Verification items for this drawing (mm, ordinates from the low corner). Give positions to 0.01 mm unless a question says otherwise; leave off trailing zeros. Order: outer loops, then holes, each group sorted by start corner. A loop starts at its lowest first (then second) coordinate and runs counter-clockwise, first axis right, second up. Notation, with made-up numbers: M 54.5,43.25 L 58.5,43.25 A23 cw 58.5,69.25 Z; hole C 12,52.5 d1. An arc over 180 degrees is marked long. Return JSON: item names as keys, results as strings. Group by question number.
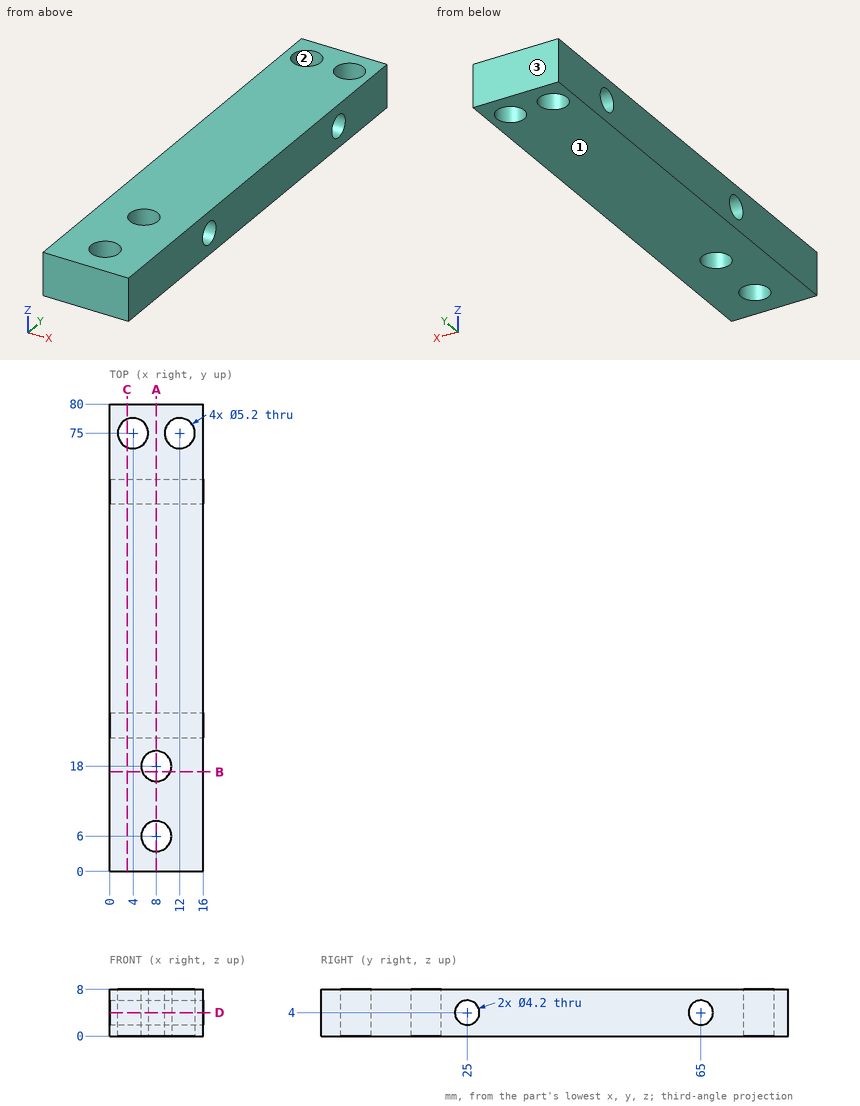
1) Sectioned sample at C-C on x = 3. Record the boundary of the cut face in (y, z).
2) Sectioned sample at D-D on z = 4. Record the boundary of the cut face in (x, y), then the cut area to 3 significant figures.
3) Release check for a two-part mould opening along Y. For the marked faces 1, 2 and 3 record: released by +Y, released by -Y, zero draft, split by the parting line, or undercut.
4) Sectioned sample at A-A on x = 8. Record the boundary of the cut face in (y, z).
5) Material ranges on line 1 along Z through (x, y) = (11.75, 25); line 2 along X through (y, z) = (73, 1.5); line 3 along Y through (x, z) = (14.75, 3.5), recorded low to high.
6) Sectioned sample at B-B on y = 17. Record the boundary of the cut face in (x, z), then the cut area to 3 significant figures.
7) Depth check by flat-ended pin: P1, Ø4, axis at x = 8, y = 6, coming from the -Z side. Enter the tip coordinate at first touch or a pass-through.
Reply:
{
 "1": {"outline": "M 0,0 L 72.6,0 L 72.6,8 L 0,8 Z; M 77.4,0 L 80,0 L 80,8 L 77.4,8 Z; hole C 25,4 d4.2; hole C 65,4 d4.2"},
 "2": {"outline": "M 0,0 L 16,0 L 16,22.9 L 0,22.9 Z; M 0,27.1 L 16,27.1 L 16,62.9 L 0,62.9 Z; M 0,67.1 L 16,67.1 L 16,80 L 0,80 Z; hole C 4,75 d5.2; hole C 8,6 d5.2; hole C 8,18 d5.2; hole C 12,75 d5.2", "area": "1,060 mm^2"},
 "3": {"face 1": "zero draft", "face 2": "undercut", "face 3": "released by +Y"},
 "4": {"outline": "M 0,0 L 3.4,0 L 3.4,8 L 0,8 Z; M 8.6,0 L 15.4,0 L 15.4,8 L 8.6,8 Z; M 20.6,0 L 80,0 L 80,8 L 20.6,8 Z; hole C 25,4 d4.2; hole C 65,4 d4.2"},
 "5": {"line 1": "0 to 1.9, 6.1 to 8", "line 2": "0 to 2.34, 5.66 to 10.34, 13.66 to 16", "line 3": "0 to 22.96, 27.04 to 62.96, 67.04 to 80"},
 "6": {"outline": "M 0,0 L 5.6,0 L 5.6,8 L 0,8 Z; M 10.4,0 L 16,0 L 16,8 L 10.4,8 Z", "area": "89.6 mm^2"},
 "7": {"P1": "through"}
}
